from build123d import *

# Parameters (mm, degrees)
BOSS_EXTRUDE1_DEPTH      = 75
BOSS_EXTRUDE1_DEPTH_BACK = 75
SKETCH3_R                = 1.6
SKETCH1_W                = 15
SKETCH1_H                = 45
FILLET1_R                = 2


with BuildPart() as part:
    # Sketch3 → Boss-Extrude1 (new, two sides: drawn at the far end of the back side and taken through both)
    with BuildSketch(Plane.XY.offset(-BOSS_EXTRUDE1_DEPTH_BACK)):
        with BuildLine():
            add(Edge.make_bspline(
                [(-96.388888889, 0), (-94.217851925, -7.513577122), (-46.388888889, 0)],
                knots=[0, 0, 0, 1, 1, 1], degree=2))
            add(Edge.make_bspline(
                [(-96.388888889, 0), (-94.217851925, 7.513577122), (-46.388888889, 0)],
                knots=[0, 0, 0, 1, 1, 1], degree=2))
        make_face()
        with Locations((-86.388888889, 0)):
            Circle(SKETCH3_R, mode=Mode.SUBTRACT)
    extrude(amount=BOSS_EXTRUDE1_DEPTH + BOSS_EXTRUDE1_DEPTH_BACK)

    # Sketch1 → Cut-Revolve1 (revolve, cut)
    with BuildSketch(Plane(origin=(0, 0, 0), x_dir=(1, 0, 0), z_dir=(0, 1, 0))):
        with Locations((-88.888888889, 0)):
            Rectangle(SKETCH1_W, SKETCH1_H)
    revolve(axis=Axis((-96.388888889, 0, -75), (0, 0, 1)), mode=Mode.SUBTRACT)

    # Fillet1
    fillet1_edges = [part.edges().sort_by_distance(p)[0] for p in [
        (-81.86563433, -3.751676562, -11.2499997),
        (-81.86563433, 3.751676562, 11.25),
    ]]
    fillet(fillet1_edges, radius=FILLET1_R)


solid = part.part
Build history of the part. All positions in model axes, mm. Coordinates: 2 decimals unless noted, no trailing zeros. Put each result on its own line as item: value.
1. Pull direction X, two halves, no side cores. Call faces 1 (the face through (-84.91, -0.61, 48.38)), 2 (the face through (-81.39, -0.02, -0.32)), 3 (the face through (-84.91, -0.61, -49.12)), 4 (the face through (-75, -1, 75)): pulls with the +X half, pulls with the -X half, needs draft (parallel to the pull), parting line crosses it, or undercut.
Answer sheet:
face 1: undercut
face 2: pulls with the -X half
face 3: undercut
face 4: needs draft
2. Probe line 1 along Z through (x, y) = (-88, -1.25); line 2 along Y through (x, z) = (-80, 48); line 3 along Y through (x, z) = (-87, -27). List the from-to ranges inside material, lowest first. Write a range as [from, to].
Answer sheet:
line 1: z = [-75, -22.5], [22.5, 75]
line 2: y = [-3.71, 3.71]
line 3: y = [-3.63, -1.48], [1.48, 3.63]
3. Drop flat-ended pins along their axis: P1, Ø8, axis at x = -75.5, z = 18, coming from the -Y side; P2, Ø1.5, axis at y = -2.5, z = -27, coming from the -X side; P3, Ø1.5, axis at x = -73, z = 29.5, coming from the +Y side. Give the stop position or say it passes through.
Answer sheet:
P1: stops at y = -3.7
P2: stops at x = -94.98
P3: stops at y = 3.38
